Could you check a few things on this drawing? It's one solid part, dimensions in mm from its lowest x, y, z. Round coordinates to 2 decimals unless told otherwise and drop trailing zeros. Order: outer loops, then holes, each group sorted by start corner. A loop starts at its lowest first (then second) coordinate and runs counter-clockwise, first axis right, second up. Notation, with made-up numbers: (69.25, 48.25) -> (73.25, 48.25) arc R20 cw to (73.25, 53.25) -> close; hole circle Ø3 at (11, -14.75). An arc over 180 degrees is marked (long way). Use a Markdown table: item, result. Add a question column.
(1) Thinking about a two-plate mould opening in X: for the marked faces 1 and 2, which applies, pulls with the +X half, pulls with the -X half, needs draft (parallel to the pull), parting line crosses it, or undercut?
(2) I'm going to push flat-ended pins straight in: P1, Ø1.5, axis at y = 23, z = 1, coming from the +X side; P2, Ø1.5, axis at y = 29.5, z = 4, coming from the -X side; P3, Ø2, axis at x = 38, z = 4.5, coming from the +Y side. Where does each tip first touch, or does it pass through?
(3) I want a section at D-D, the plane y = 38.5. Please give me the cut outline in (x, z) (3 decimals), then the cut area to 3 significant figures.
(4) If I drill on probe 1 along Y at (x, z) = (28.5, 6.5); probe 2 along X at (y, z) = (27, 5); probe 3 along X at (y, z) = (26.5, 5), over which ranges is the centre line in solid material (lowest first)?
(5) I want a section at C-C, the plane z = 3.25. Please give me the cut outline in (x, y) (3 decimals), then the cut area to 3 significant figures.
(6) I want a section at A-A, the plane y = 28. Please give me the cut outline in (x, z), then the cut area to 3 significant figures.
(7) I want a section at B-B, the plane x = 28. Please give me the cut outline in (y, z).
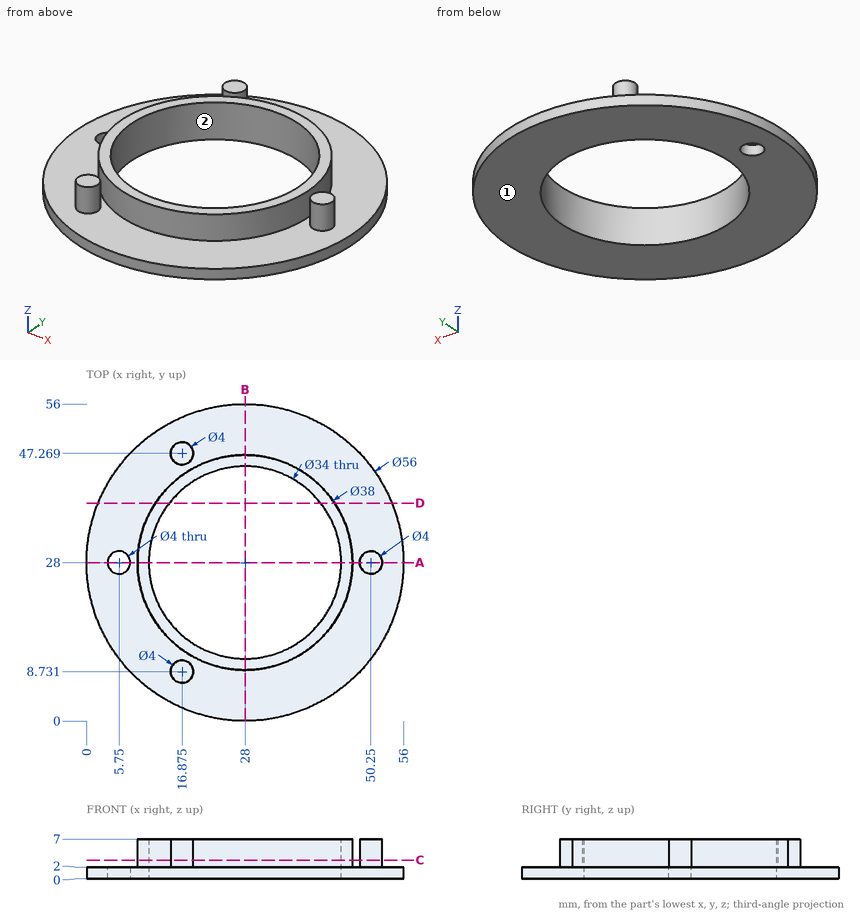
Taken from the geometry:
| question | item | result |
|---|---|---|
| 1 | face 1 | needs draft |
| 1 | face 2 | undercut |
| 2 | P1 | stops at x = 55.68 |
| 2 | P2 | stops at x = 9.01 |
| 2 | P3 | stops at y = 44.73 |
| 3 | outline | (2.043, 0) -> (14.63, 0) -> (14.63, 7) -> (12.165, 7) -> (12.165, 2) -> (2.043, 2) -> close; (41.37, 0) -> (53.957, 0) -> (53.957, 2) -> (43.835, 2) -> (43.835, 7) -> (41.37, 7) -> close |
| 3 | area | 75.0 mm2 |
| 4 | probe 1 | y = 9.01 to 11.01, 44.99 to 46.99 |
| 4 | probe 2 | x = 9.03 to 11.03, 44.97 to 46.97, 48.52 to 51.98 |
| 4 | probe 3 | x = 9.06 to 11.07, 44.93 to 46.94, 48.93 to 51.57 |
| 5 | outline | circle Ø38 at (28, 28); circle Ø4 at (16.875, 8.731); circle Ø4 at (16.875, 47.269); circle Ø4 at (50.25, 28); hole circle Ø34 at (28, 28) |
| 5 | area | 264 mm2 |
| 6 | outline | (0, 0) -> (3.75, 0) -> (3.75, 2) -> (0, 2) -> close; (7.75, 0) -> (11, 0) -> (11, 7) -> (9, 7) -> (9, 2) -> (7.75, 2) -> close; (45, 0) -> (56, 0) -> (56, 2) -> (52.25, 2) -> (52.25, 7) -> (48.25, 7) -> (48.25, 2) -> (47, 2) -> (47, 7) -> (45, 7) -> close |
| 6 | area | 76.0 mm2 |
| 7 | outline | (0, 0) -> (11, 0) -> (11, 7) -> (9, 7) -> (9, 2) -> (0, 2) -> close; (45, 0) -> (56, 0) -> (56, 2) -> (47, 2) -> (47, 7) -> (45, 7) -> close |
